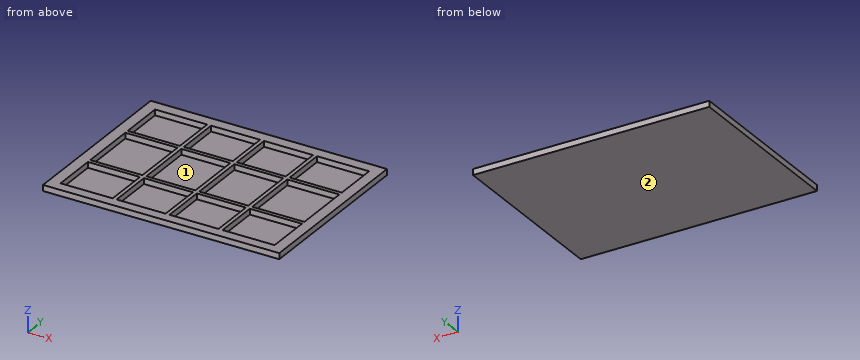
from build123d import *

# Parameters (mm, degrees)
SKETCH2_W           = 1200
SKETCH2_H           = 900
BOSS_EXTRUDE2_DEPTH = 30
SKETCH3_W           = 1087.423470631
SKETCH3_H           = 789.777232946
CUT_EXTRUDE2_DEPTH  = 29
RIB6_REACH          = 1502.3
SKETCH6_WALLS_W     = 20
SKETCH6_WALLS_H     = 3792.377172958
SKETCH6_WALLS_W_2   = 4090.023410643
SKETCH6_WALLS_H_2   = 20


with BuildPart() as part:
    # Sketch2 → Boss-Extrude2 (new body)
    with BuildSketch(Plane.XY):
        with Locations((600, 450)):
            Rectangle(SKETCH2_W, SKETCH2_H)
    extrude(amount=BOSS_EXTRUDE2_DEPTH)

    # Sketch3 → Cut-Extrude2 (cut)
    with BuildSketch(Plane.XY.offset(30)):
        with Locations((600.845585903, 447.040449341)):
            Rectangle(SKETCH3_W, SKETCH3_H)
    extrude(amount=-CUT_EXTRUDE2_DEPTH, mode=Mode.SUBTRACT)

    # Sketch6 walls → Rib6 (add, up to next)
    with BuildSketch(Plane.XY.offset(30), mode=Mode.PRIVATE) as rib6_sk1:
        with Locations((600.845585903, 447.040449341)):
            Rectangle(SKETCH6_WALLS_W, SKETCH6_WALLS_H)
    rib6_tool1 = extrude(rib6_sk1.sketch, amount=-RIB6_REACH, mode=Mode.PRIVATE) - part.part
    # Sketch6 walls → Rib6 (add, up to next)
    with BuildSketch(Plane.XY.offset(30), mode=Mode.PRIVATE) as rib6_sk2:
        with Locations((331.949268904, 447.040449341)):
            Rectangle(SKETCH6_WALLS_W, SKETCH6_WALLS_H)
    rib6_tool2 = extrude(rib6_sk2.sketch, amount=-RIB6_REACH, mode=Mode.PRIVATE) - part.part
    # Sketch6 walls → Rib6 (add, up to next)
    with BuildSketch(Plane.XY.offset(30), mode=Mode.PRIVATE) as rib6_sk3:
        with Locations((600.845585903, 603.473841306)):
            Rectangle(SKETCH6_WALLS_W_2, SKETCH6_WALLS_H_2)
    rib6_tool3 = extrude(rib6_sk3.sketch, amount=-RIB6_REACH, mode=Mode.PRIVATE) - part.part
    # Sketch6 walls → Rib6 (add, up to next)
    with BuildSketch(Plane.XY.offset(30), mode=Mode.PRIVATE) as rib6_sk4:
        with Locations((869.741902901, 447.040449341)):
            Rectangle(SKETCH6_WALLS_W, SKETCH6_WALLS_H)
    rib6_tool4 = extrude(rib6_sk4.sketch, amount=-RIB6_REACH, mode=Mode.PRIVATE) - part.part
    # Sketch6 walls → Rib6 (add, up to next)
    with BuildSketch(Plane.XY.offset(30), mode=Mode.PRIVATE) as rib6_sk5:
        with Locations((600.845585903, 290.607057376)):
            Rectangle(SKETCH6_WALLS_W_2, SKETCH6_WALLS_H_2)
    rib6_tool5 = extrude(rib6_sk5.sketch, amount=-RIB6_REACH, mode=Mode.PRIVATE) - part.part
    add(rib6_tool1.solids().sort_by_distance((600.845585903, 447.040449341, 30))[0])
    add(rib6_tool2.solids().sort_by_distance((331.949268904, 447.040449341, 30))[0])
    add(rib6_tool3.solids().sort_by_distance((600.845585903, 603.473841306, 30))[0])
    add(rib6_tool4.solids().sort_by_distance((869.741902901, 447.040449341, 30))[0])
    add(rib6_tool5.solids().sort_by_distance((600.845585903, 290.607057376, 30))[0])


solid = part.part
Read the model definition and answer for the solid it produces. Units are mm, in the model's axes. Face numbers are marked on the shaded views. Give positions to 0.01 mm unless a question says otherwise; leave off trailing zeros. Loops run counter-clockwise (first coordinate to the right, second up) from the corner with the lowest first, then second, coordinate; pieces in that order, holes last. Notation, with made-up numbers: (-7, -25.5) -> (26, -25.5) arc R20 ccw to (26, -3.5) -> close; hole circle Ø7 at (-18.5, -35). An arc over 180 degrees is marked (long way). Use a Markdown table: item, result.
Q1. Find the intervals of material crossed by line 1 along Y through (x, z) = (700.5, 9.25); line 2 along X through (y, z) = (131, 24.75); line 3 along Z through (x, y) = (141, 272), in increasing order.
Solved:
| item | result |
|---|---|
| line 1 | y = 0 to 52.15, 280.61 to 300.61, 593.47 to 613.47, 841.93 to 900 |
| line 2 | x = 0 to 57.13, 321.95 to 341.95, 590.85 to 610.85, 859.74 to 879.74, 1144.56 to 1200 |
| line 3 | z = 0 to 1 |
Q2. Section B-B, the plane x = 573 is taken. Determine the outline of the cut face in (y, z), then the cut area to 3 significant figures.
Solved:
| item | result |
|---|---|
| outline | (0, 0) -> (900, 0) -> (900, 30) -> (841.93, 30) -> (841.93, 1) -> (613.47, 1) -> (613.47, 30) -> (593.47, 30) -> (593.47, 1) -> (300.61, 1) -> (300.61, 30) -> (280.61, 30) -> (280.61, 1) -> (52.15, 1) -> (52.15, 30) -> (0, 30) -> close |
| area | 5,260 mm^2 |
Q3. Determine the mould class of the marked faces 1 and 2 for opening direction X: pulls with the +X half, pulls with the -X half, needs draft (parallel to the pull), parting line crosses it, or undercut.
Solved:
| item | result |
|---|---|
| face 1 | undercut |
| face 2 | needs draft |
Q4. This flat-tipped pin is pushed along its axis until it touches: pin 1 (8 mm diameter, centred on x = 194, y = 398.5, fed in from +Z). Where does it stop, or does it pass through?
Solved:
| item | result |
|---|---|
| pin 1 | stops at z = 1 |
Q5. Section A-A, the plane y = 103 is taken. Determine the outline of the cut face in (x, z), then the cut area to 3 significant figures.
Solved:
| item | result |
|---|---|
| outline | (0, 0) -> (1200, 0) -> (1200, 30) -> (1144.56, 30) -> (1144.56, 1) -> (879.74, 1) -> (879.74, 30) -> (859.74, 30) -> (859.74, 1) -> (610.85, 1) -> (610.85, 30) -> (590.85, 30) -> (590.85, 1) -> (341.95, 1) -> (341.95, 30) -> (321.95, 30) -> (321.95, 1) -> (57.13, 1) -> (57.13, 30) -> (0, 30) -> close |
| area | 6,200 mm^2 |
Q6. Section C-C, the plane z = 6 is taken. Count the separate pieces of the cut face and the enclosed holes in it, then the cut area to 3 significant figures.
Solved:
| item | result |
|---|---|
| separate pieces | 1 |
| enclosed holes | 12 |
| area | 310,000 mm^2 |
